from build123d import *

# Parameters (mm, degrees)
F0_W     = 80
F0_H     = 50
F0_R     = 2.5
F0_R_2   = 5.5
F1_DEPTH = 12
F2_R     = 8
F2_R_2   = 5.5
F3_DEPTH = 5


with BuildPart() as f1:
    # F0 (on Front) → F1 (new body)
    with BuildSketch(Plane.XZ):
        Rectangle(F0_W, F0_H)
        with Locations((-10, -15)):
            Circle(F0_R, mode=Mode.SUBTRACT)
        with Locations((10, -15)):
            Circle(F0_R, mode=Mode.SUBTRACT)
        with Locations((-30, 5)):
            Circle(F0_R, mode=Mode.SUBTRACT)
        with Locations((0, 7)):
            Circle(F0_R_2, mode=Mode.SUBTRACT)
        with Locations((30, 5)):
            Circle(F0_R, mode=Mode.SUBTRACT)
    extrude(amount=F1_DEPTH)

    # F2 (on face) → F3 (cut)
    with BuildSketch(Plane.XZ.offset(12)):
        with Locations((0, 7)):
            Circle(F2_R)
        with Locations((0, 7)):
            Circle(F2_R_2, mode=Mode.SUBTRACT)
    extrude(amount=-F3_DEPTH, mode=Mode.SUBTRACT)


solid = f1.part
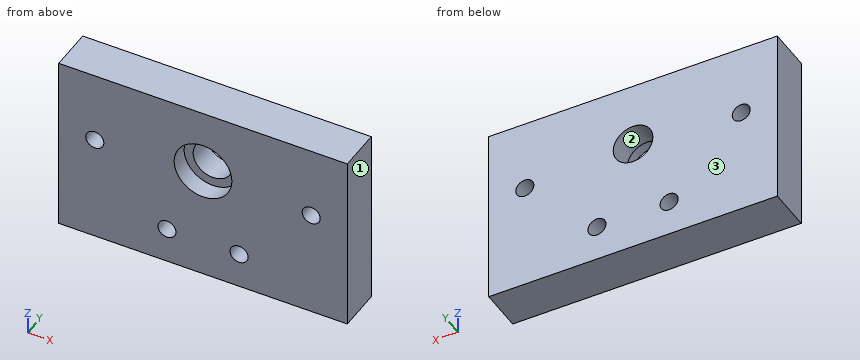
Build history of the part. All positions in model axes, mm. Face numbers are marked on the shaded views. Round coordinates to 2 decimals unless told otherwise and drop trailing zeros. Loops run counter-clockwise (first coordinate to the right, second up) from the corner with the lowest first, then second, coordinate; pieces in that order, holes last. Notation, with made-up numbers: (86, 62.5) -> (121, 62.5) arc R17 cw to (121, 88.5) -> close; hole circle Ø5 at (-21.5, -35.75). An arc over 180 degrees is marked (long way). Answer in a Markdown table with one row per item.
Item 1: Saw through at D-D (z = 9.5). Write the cut outline in (x, y).
Answers below:
| item | result |
|---|---|
| outline | (-40, -12) -> (-7.6, -12) -> (-7.6, -7) -> (-4.9, -7) -> (-4.9, 0) -> (-40, 0) -> close; (4.9, -7) -> (7.6, -7) -> (7.6, -12) -> (40, -12) -> (40, 0) -> (4.9, 0) -> close |
Item 2: Saw through at C-C (y = -10.5). Write the cut outline in (x, z).
Answers below:
| item | result |
|---|---|
| outline | (-40, -25) -> (40, -25) -> (40, 25) -> (-40, 25) -> close; hole circle Ø5 at (-30, 5); hole circle Ø5 at (-10, -15); hole circle Ø16 at (0, 7); hole circle Ø5 at (10, -15); hole circle Ø5 at (30, 5) |
Item 3: Saw through at A-A (x = -30). Write the cut outline in (y, z), and give its area (3 significant figures).
Answers below:
| item | result |
|---|---|
| outline | (-12, -25) -> (0, -25) -> (0, 2.5) -> (-12, 2.5) -> close; (-12, 7.5) -> (0, 7.5) -> (0, 25) -> (-12, 25) -> close |
| area | 540 mm² |
Item 4: Saw through at B-B (z = -15). Write the cut outline in (x, y), and give its area (3 significant figures).
Answers below:
| item | result |
|---|---|
| outline | (-40, -12) -> (-12.5, -12) -> (-12.5, 0) -> (-40, 0) -> close; (-7.5, -12) -> (7.5, -12) -> (7.5, 0) -> (-7.5, 0) -> close; (12.5, -12) -> (40, -12) -> (40, 0) -> (12.5, 0) -> close |
| area | 840 mm² |
Item 5: Mould opens along X. For the marked faces 1, 2 and 3 say: +X half, -X half, draft (parallel to the pull), parting line (faces both ways), or undercut.
Answers below:
| item | result |
|---|---|
| face 1 | +X half |
| face 2 | undercut |
| face 3 | draft |
Item 6: Drill centre lines: L1, parallel to Z at x = -10, y = -4.5; L2, parallel to Z at x = -30, y = -3.5; L3, parallel to X at y = -4.5, z = -14. Where is each one in solid material? Low to high. Write a range as [from, to].
Answers below:
| item | result |
|---|---|
| L1 | z = [-25, -17.5], [-12.5, 25] |
| L2 | z = [-25, 2.5], [7.5, 25] |
| L3 | x = [-40, -12.29], [-7.71, 7.71], [12.29, 40] |
Item 7: Pin check, flat tip, straight feed: pin 1 (12.5 mm diameter, centred on x = 0, z = 7, fed in from -Y). Stop position of the tip, or through.
Answers below:
| item | result |
|---|---|
| pin 1 | stops at y = -7 |
